Can you work these out from the model? Positions are in its coordinate system, mm. Face numbers are marked on the shaded views. A direction names the side the tool comes from. Round coordinates to 2 decimals unless told otherwise and drop trailing zeros. Loops run counter-clockwise (first coordinate to the right, second up) from the corner with the lowest first, then second, coordinate; pieces in that order, holes last.
(1) I want a section at B-B on z = 0. Write out the boundary of the cut face in (x, y), plus the area to 3 significant figures.
(2) I want a section at C-C on y = -114. Write out the boundary of the cut face in (x, z), plus the area to 3 significant figures.
(3) If I drill on line 1 along Y through (x, z) = (-17.5, 5); line 2 along Y through (x, z) = (-6, -4.5); line 3 along Z through (x, y) = (3, 10), over which ranges is the centre line in solid material (lowest first)?
(4) I want a section at A-A on x = 0. Write out the boundary of the cut face in (y, z).
(5) I want a section at D-D on z = 11. Write out the boundary of the cut face in (x, y), plus the area to 3 significant figures.
(6) Which directions (+Z, -Z, +X, -X, +Y, -Y) give clear straight access to the entire face, cutting with the end or side of a thin tool? Please do the marked faces 1, 2 and 3.
(7) Will these pins go through, and if not, where does the flat tip stop? pin 1 Ø1 at (x, y) = (8, -35) entering from +Z; pin 2 Ø6 at (y, z) = (-92.5, -2) entering from +X; pin 3 Ø12 at (y, z) = (-95.5, 0) entering from -X.
(8) Thinking about a two-plate mould opening in Z: for the marked faces 4 and 5, which applies, released by +Z, released by -Z, zero draft, split by the parting line, or undercut?
from build123d import *

# Parameters (mm, degrees)
F0_R     = 20
F1_DEPTH = 60
F3_R     = 15
F4_DEPTH = 45
F2_R     = 15
F5_DEPTH = 45
F6_R     = 6.5
F7_DEPTH = 30


with BuildPart() as f1:
    # F0 (on Front) → F1 (new body)
    with BuildSketch(Plane.XZ):
        Circle(F0_R)
    extrude(amount=F1_DEPTH)

    # F3 (on face) → F4 (join)
    with BuildSketch(Plane(origin=(0, 0, 0), x_dir=(-1, 0, 0), z_dir=(0, 1, 0))):
        Circle(F3_R)
    extrude(amount=F4_DEPTH)

    # F2 (on face) → F5 (join)
    with BuildSketch(Plane.XZ.offset(60)):
        Circle(F2_R)
    extrude(amount=F5_DEPTH)

    # F6 (on face) → F7 (join)
    with BuildSketch(Plane.XZ.offset(105)):
        Circle(F6_R)
    extrude(amount=F7_DEPTH)


solid = f1.part
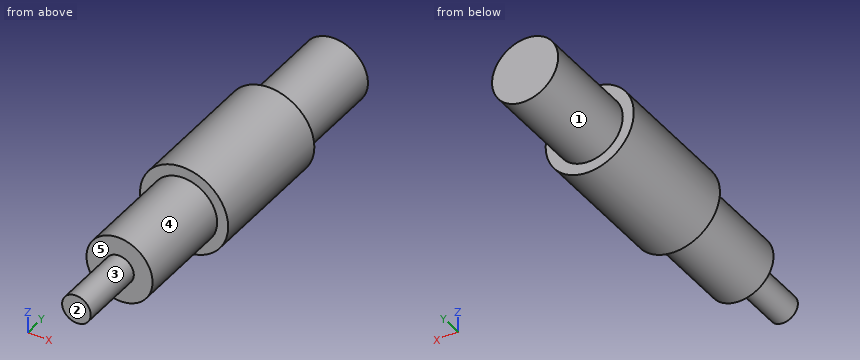
Filled sheet:
1. outline: (-20, -60) - (-15, -60) - (-15, -105) - (-6.5, -105) - (-6.5, -135) - (6.5, -135) - (6.5, -105) - (15, -105) - (15, -60) - (20, -60) - (20, 0) - (15, 0) - (15, 45) - (-15, 45) - (-15, 0) - (-20, 0) - close
1. area: 5,490 mm2
2. outline: circle Ø13 at (0, 0)
2. area: 133 mm2
3. line 1: y = -60 to 0
3. line 2: y = -105 to 45
3. line 3: z = -14.7 to 14.7
4. outline: (-135, -6.5) - (-105, -6.5) - (-105, -15) - (-60, -15) - (-60, -20) - (0, -20) - (0, -15) - (45, -15) - (45, 15) - (0, 15) - (0, 20) - (-60, 20) - (-60, 15) - (-105, 15) - (-105, 6.5) - (-135, 6.5) - close
5. outline: (-16.7, -60) - (-10.2, -60) - (-10.2, -105) - (10.2, -105) - (10.2, -60) - (16.7, -60) - (16.7, 0) - (10.2, 0) - (10.2, 45) - (-10.2, 45) - (-10.2, 0) - (-16.7, 0) - close
5. area: 3,840 mm2
6. face 1: +Y
6. face 2: +Z, -Z, +X, -X, -Y
6. face 3: -Y
7. pin 1: stops at z = 18.54
7. pin 2: stops at x = 15
7. pin 3: stops at x = -15
8. face 4: split by the parting line
8. face 5: zero draft
